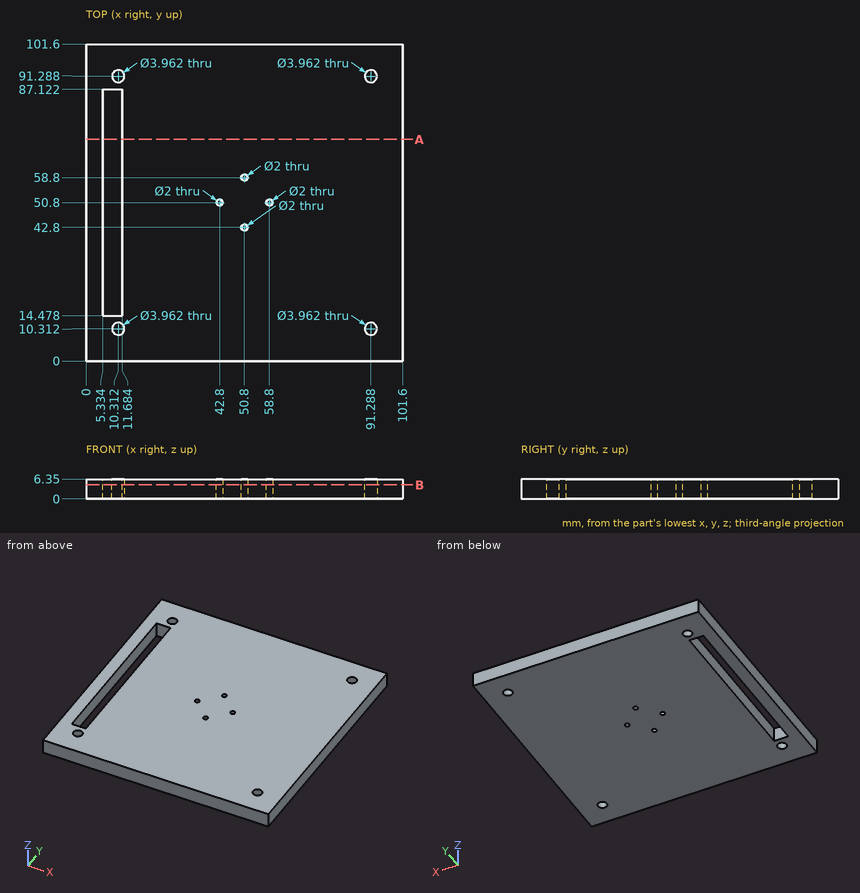
Answer from the drawing. Dimensions are ordinates in mm from the lowest x, y and z of the part. Give positions to 0.01 mm unless a question says otherwise; leave off trailing zeros. Write each loop counter-clockwise with the first axis right and the second up, starting at its lowest first coordinate (ties: lowest second). Pieces come first, ordered by that corner, then holes. Notation, with made-up numbers: (23, 37.25) - (60, 37.25) arc R14 ccw to (60, 44.25) - close; hole circle Ø5 at (-0.5, 7.5). An arc over 180 degrees is marked (long way). One line per item, written item: value. Start each with the question number.
1. Find section A-A (y = 71). Write down the section's boundary in (x, z).
2. Find section B-B (z = 4.5). State how many separate pieces and enclosed holes the cut face has, then the cut area to 3 significant figures.
3. Given pin 1 (1.8 mm diameter, centred on x = 58.8, y = 50.8, fed in from -Z), flat-ended and moving along its own axis, determine where the tip first touches the part or whether it passes through.
4. Consider probe 1 along X at (y, z) = (10.5, 1.75) (1 decimal); probe 2 along X at (y, z) = (46.5, 5.5); probe 3 along Y at (x, z) = (42.8, 3). Determine where each line is inside the solid, lowest interval first.
Geometry results:
1. outline: (0, 0) - (5.33, 0) - (5.33, 6.35) - (0, 6.35) - close; (11.68, 0) - (101.6, 0) - (101.6, 6.35) - (11.68, 6.35) - close
2. separate pieces: 1
2. enclosed holes: 9
2. area: 9,800 mm2
3. pin 1: through
4. probe 1: 0 to 8.3, 12.3 to 89.3, 93.3 to 101.6
4. probe 2: 0 to 5.33, 11.68 to 101.6
4. probe 3: 0 to 49.8, 51.8 to 101.6
